```python
from build123d import *

# Parameters (mm, degrees)
EXTRUDE_1_DEPTH                  = 2
CUT_EXTRUDE_1_DEPTH              = 57.603886792
EXTRUDE_2_DEPTH                  = 6
EXTRUDE_3_DEPTH                  = 6
SKETCH_5_W                       = 1.65
SKETCH_5_H                       = 32
HOLE_WIZARD_3_3_3_3_1_AT_2_COUNT = 2
HOLE_WIZARD_3_3_3_3_1_AT_2_PITCH = 46
HOLE_WIZARD_3_3_3_3_2_D          = 3.3
HOLE_WIZARD_3_3_3_3_2_DEPTH      = 52
HOLE_WIZARD_3_0_3_1_D            = 3
HOLE_WIZARD_3_0_3_1_DEPTH        = 8
FILLET_1_R                       = 0.5
FILLET_2_R                       = 2


with BuildPart() as part:
    # 草图1 → 凸台-拉伸1 (new body)
    with BuildSketch(Plane(origin=(62, 0, 0), x_dir=(0, 0, -1), z_dir=(1, 0, 0))):
        with BuildLine():
            Line((20.615528128, 40), (-20.615528128, 40))
            ThreePointArc((-20.615528128, 40), (-31.819805153, 31.819805153), (-40, 20.615528128))
            Line((-40, 20.615528128), (-40, -20.615528128))
            ThreePointArc((-40, -20.615528128), (-31.819805153, -31.819805153), (-20.615528128, -40))
            Line((-20.615528128, -40), (20.615528128, -40))
            ThreePointArc((20.615528128, -40), (31.819805153, -31.819805153), (40, -20.615528128))
            Line((40, -20.615528128), (40, 20.615528128))
            ThreePointArc((40, 20.615528128), (31.819805153, 31.819805153), (20.615528128, 40))
        make_face()
    extrude(amount=-EXTRUDE_1_DEPTH)

    # 草图2 → 切除-拉伸1 (cut, through all)
    with BuildSketch(Plane.ZY.offset(-60)):
        with BuildLine():
            Line((5, -28.057975693), (5, -19.364916731))
            ThreePointArc((5, -19.364916731), (14.142135624, -14.142135624), (19.364916731, -5))
            Line((19.364916731, -5), (28.057975693, -5))
            ThreePointArc((28.057975693, -5), (28.5, 0), (28.057975693, 5))
            Line((28.057975693, 5), (19.364916731, 5))
            ThreePointArc((19.364916731, 5), (14.142135624, 14.142135624), (5, 19.364916731))
            Line((5, 19.364916731), (5, 28.057975693))
            ThreePointArc((5, 28.057975693), (0, 28.5), (-5, 28.057975693))
            Line((-5, 28.057975693), (-5, 19.364916731))
            ThreePointArc((-5, 19.364916731), (-14.142135624, 14.142135624), (-19.364916731, 5))
            Line((-19.364916731, 5), (-28.057975693, 5))
            ThreePointArc((-28.057975693, 5), (-28.5, 0), (-28.057975693, -5))
            Line((-28.057975693, -5), (-19.364916731, -5))
            ThreePointArc((-19.364916731, -5), (-14.142135624, -14.142135624), (-5, -19.364916731))
            Line((-5, -19.364916731), (-5, -28.057975693))
            ThreePointArc((-5, -28.057975693), (0, -28.5), (5, -28.057975693))
        make_face()
    extrude(amount=-CUT_EXTRUDE_1_DEPTH, mode=Mode.SUBTRACT)

    # 草图3 → 凸台-拉伸2 (add)
    with BuildSketch(Plane.ZY.offset(-60)):
        Polygon((12, -16), (12, -40), (-12, -40), (-12, -16), (-8, -16), (-8, -38), (8, -38), (8, -16), align=None)
    extrude(amount=EXTRUDE_2_DEPTH)

    # 草图4 → 凸台-拉伸3 (add)
    with BuildSketch(Plane.ZY.offset(-60)):
        Polygon((12, 16), (8, 16), (8, 38), (-8, 38), (-8, 16), (-12, 16), (-12, 40), (12, 40), align=None)
    extrude(amount=EXTRUDE_3_DEPTH)

    # 草图5 → Ø3.3 (3.3) 直径孔1 (revolve, cut)
    with BuildSketch(Plane(origin=(57, -23, 8), x_dir=(0, 1, 0), z_dir=(1, 0, 0))):
        with Locations((0.825, 16)):
            Rectangle(SKETCH_5_W, SKETCH_5_H)
    hole_wizard_3_3_3_3_1 = revolve(axis=Axis((57, -23, 1.65), (0, 0, 1)), mode=Mode.SUBTRACT)

    # Ø3.3 (3.3) 直径孔1 at 2: Ø3.3 (3.3) 直径孔1 ×2
    with Locations(*[(0, i * HOLE_WIZARD_3_3_3_3_1_AT_2_PITCH, 0) for i in range(1, HOLE_WIZARD_3_3_3_3_1_AT_2_COUNT)]):
        add(hole_wizard_3_3_3_3_1, mode=Mode.SUBTRACT)

    # Ø3.3 (3.3) 直径孔2
    with Locations(Plane(origin=(0, 0, -12), x_dir=(-1, 0, 0), z_dir=(0, 0, -1))):
        with Locations((-57, -23), (-57, 23)):
            Hole(HOLE_WIZARD_3_3_3_3_2_D / 2, depth=HOLE_WIZARD_3_3_3_3_2_DEPTH)

    # Ø3.0 (3) 直径孔1
    with Locations(Plane(origin=(62, 0, 0), x_dir=(0, 0, -1), z_dir=(1, 0, 0))):
        with Locations((0, 32), (-22.627416998, 22.627416998), (-32, 0), (-22.627416998, -22.627416998), (0, -32), (22.627416998, -22.627416998), (32, 0), (22.627416998, 22.627416998)):
            Hole(HOLE_WIZARD_3_0_3_1_D / 2, depth=HOLE_WIZARD_3_0_3_1_DEPTH)

    # 圆角1
    # the kernel refuses this fillet: 0.5 mm, written as the material it adds along each edge
    with BuildSketch(Plane(origin=(61.25, 38, -8), x_dir=(0, 0, 1), z_dir=(-1, 0, 0)), Plane(origin=(61.25, 38, 8), x_dir=(0, -1, 0), z_dir=(-1, 0, 0)), Plane(origin=(61.25, -38, 8), x_dir=(0, 0, -1), z_dir=(-1, 0, 0)), Plane(origin=(61.25, -38, -8), x_dir=(0, 1, 0), z_dir=(-1, 0, 0))) as fillet_1_piece_1:
        with BuildLine():
            CenterArc((FILLET_1_R, -FILLET_1_R), FILLET_1_R, 90, 90)
            Line((0, -FILLET_1_R), (0, 0))
            Line((0, 0), (FILLET_1_R, 0))
        make_face()
    extrude(amount=7.25)
    # the kernel refuses this fillet: 0.5 mm, written as the material it takes off along each edge
    with BuildSketch(Plane(origin=(60, 16, 12), x_dir=(0, 1, 0), z_dir=(-1, 0, 0)), Plane(origin=(60, -16, -12), x_dir=(0, -1, 0), z_dir=(-1, 0, 0))) as fillet_1_2_piece_1:
        with BuildLine():
            CenterArc((FILLET_1_R, FILLET_1_R), FILLET_1_R, 180, 90)
            Line((0, FILLET_1_R), (0, 0))
            Line((0, 0), (FILLET_1_R, 0))
        make_face()
    extrude(amount=7.25, mode=Mode.SUBTRACT)
    with BuildSketch(Plane(origin=(60, 16, -12), x_dir=(0, 1, 0), z_dir=(-1, 0, 0)), Plane(origin=(60, -16, 12), x_dir=(0, -1, 0), z_dir=(-1, 0, 0))) as fillet_1_2_piece_2:
        with BuildLine():
            CenterArc((FILLET_1_R, -FILLET_1_R), FILLET_1_R, 90, 90)
            Line((0, -FILLET_1_R), (0, 0))
            Line((0, 0), (FILLET_1_R, 0))
        make_face()
    extrude(amount=7.25, mode=Mode.SUBTRACT)
    with BuildSketch(Plane(origin=(61.25, 16, -8), x_dir=(0, 0, -1), z_dir=(-1, 0, 0)), Plane(origin=(61.25, -16, 8), x_dir=(0, 0, 1), z_dir=(-1, 0, 0))) as fillet_1_2_piece_3:
        with BuildLine():
            CenterArc((FILLET_1_R, -FILLET_1_R), FILLET_1_R, 90, 90)
            Line((0, -FILLET_1_R), (0, 0))
            Line((0, 0), (FILLET_1_R, 0))
        make_face()
    extrude(amount=8.5, mode=Mode.SUBTRACT)
    with BuildSketch(Plane(origin=(61.25, 16, 8), x_dir=(0, 0, 1), z_dir=(-1, 0, 0)), Plane(origin=(61.25, -16, -8), x_dir=(0, 0, -1), z_dir=(-1, 0, 0))) as fillet_1_2_piece_4:
        with BuildLine():
            CenterArc((FILLET_1_R, FILLET_1_R), FILLET_1_R, 180, 90)
            Line((0, FILLET_1_R), (0, 0))
            Line((0, 0), (FILLET_1_R, 0))
        make_face()
    extrude(amount=8.5, mode=Mode.SUBTRACT)

    # 圆角2
    fillet_2_edges = [part.edges().sort_by_distance(p)[0] for p in [
        (61, -28.057975693, 5),
        (61, -28.057975693, -5),
        (61, -19.364916731, -5),
        (61, -5, -19.364916731),
        (61, -5, -28.057975693),
        (61, 5, -28.057975693),
        (61, 5, -19.364916731),
        (61, 19.364916731, -5),
        (61, 28.057975693, -5),
        (61, 28.057975693, 5),
        (61, 19.364916731, 5),
        (61, 5, 19.364916731),
        (61, 5, 28.057975693),
        (61, -5, 28.057975693),
        (61, -5, 19.364916731),
        (61, -19.364916731, 5),
    ]]
    fillet(fillet_2_edges, radius=FILLET_2_R)


solid = part.part
```
Design review of the part built by this model. Coordinates are the model's own, in mm. A direction names the side the tool comes from. Coordinates: 2 decimals unless noted, no trailing zeros. Order: outer loops, then holes, each group sorted by start corner. A loop starts at its lowest first (then second) coordinate and runs counter-clockwise, first axis right, second up.
1) Take a section at A-A, the plane y = 0. Give the boundary of the cut face in (x, z).
2) Wall thickness on line 1 along Z through (x, y) = (59.5, -32); line 2 along Y through (x, z) = (55.25, -10); line 3 along Y through (x, z) = (57, -10): over which ranges is each line inside the solid? List them lowest first.
3) Clearance check with flat-ended pins moving along their axes: pin 1 (3 mm diameter, centred on x = 56.5, y = -24.5, fed in from +Z); pin 2 (1.6 mm diameter, centred on x = 60.5, z = 23, fed in from -Y); pin 3 (1.8 mm diameter, centred on x = 56, y = 23, fed in from -Z). State where each tip first meets the part, or that it passes through.
4) Mouldability with a two-part tool opening along Y and no side actions: class faces 1 (the cylindrical face through (61.01, 19.7, 5.37)), 2 (the flat face through (60, 17, 10)), 3 (the cylindrical face through (61.01, -31.68, 31.96)), 4 (the flat face through (57, -28, -12)) as +Y half, -Y half, draft (parallel to the pull), parting line (faces both ways), or undercut.
5) Take a section at C-C, the plane y = 12.5. Give the boundary of the cut face in (x, z), and give its area (4 significant figures).
6) For faces 5 (the cylindrical face through (61.014, -27.677, -4.478)), 6 (the cylindrical face through (60.986, -14.233, 14.05)), 7 (the flat face through (57, -16, -10)), list the 3-axis set-ups (+Z, -Z, +X, -X, +Y, -Y) from which the entire face can be reached by the end or side of a thin tool; tool diameter is ignored.
7) Take a section at D-D, the plane z = 14. Give the boundary of the cut face in (x, y), and give its area (3 significant figures).
8) Take a section at B-B, the plane z = 0. Give the boundary of the cut face in (x, y), and give its area (3 significant figures).
Returned:
1. outline: (60, -40) - (62, -40) - (62, -33.5) - (60, -33.5) - close; (60, -30.5) - (62, -30.5) - (62, -28.5) - (60, -28.5) - close; (60, 28.5) - (62, 28.5) - (62, 30.5) - (60, 30.5) - close; (60, 33.5) - (62, 33.5) - (62, 40) - (60, 40) - close
2. line 1: z = -12 to -8, 8 to 12
2. line 2: y = -40 to -16, 16 to 40
2. line 3: y = -40 to -24.65, -21.35 to -16, 16 to 21.35, 24.65 to 40
3. pin 1: stops at z = 12
3. pin 2: stops at y = -39.14
3. pin 3: stops at z = -12
4. face 1: undercut
4. face 2: undercut
4. face 3: -Y half
4. face 4: draft
5. outline: (60, -40) - (62, -40) - (62, -15.61) - (60, -15.61) - close; (60, 15.61) - (62, 15.61) - (62, 40) - (60, 40) - close
5. area: 97.55 mm2
6. face 5: +X, -X
6. face 6: +X
6. face 7: +Z, -Z, +X, -X
7. outline: (60, -40) - (62, -40) - (62, -14.28) - (60, -14.28) - close; (60, 14.28) - (62, 14.28) - (62, 40) - (60, 40) - close
7. area: 103 mm2
8. outline: (54, -40) - (62, -40) - (62, -33.5) - (60, -33.5) - (60, -38) - (54, -38) - close; (54, 38) - (60, 38) - (60, 33.5) - (62, 33.5) - (62, 40) - (54, 40) - close; (60, -30.5) - (62, -30.5) - (62, -28.5) - (60, -28.5) - close; (60, 28.5) - (62, 28.5) - (62, 30.5) - (60, 30.5) - close
8. area: 58.0 mm2
